Work out the finished part from the listing and answer in its coordinate system (mm). Face numbers are marked on the shaded views. A direction names the side the tool comes from. Round coordinates to 2 decimals unless told otherwise and drop trailing zeros. Write each loop counter-clockwise with the first axis right and the second up, starting at its lowest first coordinate (ties: lowest second). Pieces come first, ordered by that corner, then holes. Notation, with made-up numbers: M -12.75,55.5 L 4.25,55.5 A23 ccw 4.25,87.5 Z; hole C -32.75,-35 d8. An arc over 180 degrees is marked long. Answer in a Markdown table with one row per item.
```python
from build123d import *

# Parameters (mm, degrees)
SKETCH_W     = 100
SKETCH_H     = 70
PAD_DEPTH    = 15
PAD001_DEPTH = 10
POCKET_DEPTH = 5


with BuildPart() as part:
    # Sketch → Pad (new body)
    with BuildSketch(Plane.XY):
        Rectangle(SKETCH_W, SKETCH_H)
    extrude(amount=PAD_DEPTH)

    # Sketch001 (on Face6 of Pad) → Pad001 (join)
    with BuildSketch(Plane.XY.offset(15)):
        with BuildLine():
            Line((-37.5, -18), (-22.5, -18))
            ThreePointArc((-22.5, -18), (-16.843146, -15.656854), (-14.5, -10))
            Line((-14.5, -10), (-14.5, 10))
            ThreePointArc((-14.5, 10), (-16.843146, 15.656854), (-22.5, 18))
            Line((-22.5, 18), (-37.5, 18))
            ThreePointArc((-37.5, 18), (-43.156854, 15.656854), (-45.5, 10))
            Line((-45.5, 10), (-45.5, -10))
            ThreePointArc((-45.5, -10), (-43.156854, -15.656854), (-37.5, -18))
        make_face()
        with BuildLine():
            Line((-37.5, -15), (-22.5, -15))
            ThreePointArc((-22.5, -15), (-18.964466, -13.535534), (-17.5, -10))
            Line((-17.5, -10), (-17.5, 10))
            ThreePointArc((-17.5, 10), (-18.964466, 13.535534), (-22.5, 15))
            Line((-22.5, 15), (-37.5, 15))
            ThreePointArc((-37.5, 15), (-41.035534, 13.535534), (-42.5, 10))
            Line((-42.5, 10), (-42.5, -10))
            ThreePointArc((-42.5, -10), (-41.035534, -13.535534), (-37.5, -15))
        make_face(mode=Mode.SUBTRACT)
    pad001 = extrude(amount=PAD001_DEPTH)

    # Sketch002 (on Face5 of Pad001) → Pocket (cut)
    with BuildSketch(Plane.XY.offset(15)):
        Polygon((-25, 0), (-27.5, 4.330127), (-32.5, 4.330127), (-35, 0), (-32.5, -4.330127), (-27.5, -4.330127), align=None)
    pocket = extrude(amount=-POCKET_DEPTH, mode=Mode.SUBTRACT)

    # Mirrored: Pad001, Pocket across Sketch001 V_Axis
    add(pad001.mirror(Plane(origin=(0, 0, 15), x_dir=(0, 0, 1), z_dir=(1, 0, 0))))
    add(pocket.mirror(Plane(origin=(0, 0, 15), x_dir=(0, 0, 1), z_dir=(1, 0, 0))), mode=Mode.SUBTRACT)


solid = part.part
```
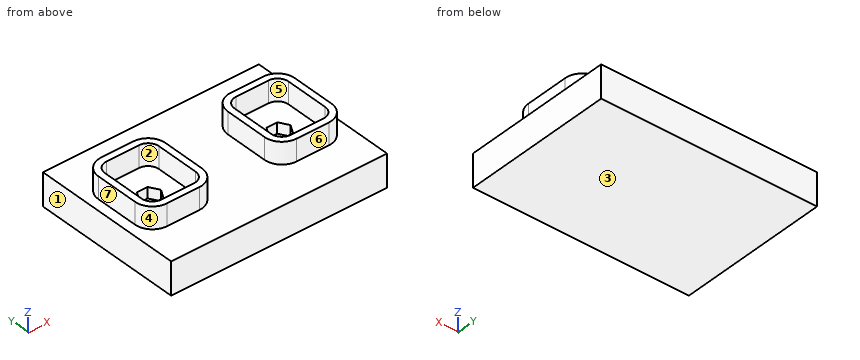
1. Given pin 1 (8 mm diameter, centred on y = -5, z = 18.5, fed in from -X); pin 2 (5 mm diameter, centred on x = -13.5, y = 16, fed in from +Z); pin 3 (3 mm diameter, centred on y = -15.5, z = 21.5, fed in from -X); pin 4 (8 mm diameter, centred on y = 4, z = 19.5, fed in from -X), each flat-ended and moving along its own axis, determine where each tip first touches the part or whether it passes through.
Calculated:
| item | result |
|---|---|
| pin 1 | stops at x = -50 |
| pin 2 | stops at z = 15 |
| pin 3 | stops at x = -44.43 |
| pin 4 | stops at x = -45.5 |
2. A tool of negligible diameter and unlimited length cuts with its end or side. For the marked faces 4, 5, 6 and 7, from which of +Z, -Z, +X, -X, +Y, -Y can it reach the whole face along a straight path? Write none if from no direction.
Calculated:
| item | result |
|---|---|
| face 4 | +Z, -X, -Y |
| face 5 | +Z |
| face 6 | +Z, +X, -X, -Y |
| face 7 | +Z, -X, +Y, -Y |
3. The part is cut by section D-D (x = 21.5). Determine the outline of the cut face in (y, z).
Calculated:
| item | result |
|---|---|
| outline | M -35,0 L 35,0 L 35,15 L 17.94,15 L 17.94,25 L 14.9,25 L 14.9,15 L -14.9,15 L -14.9,25 L -17.94,25 L -17.94,15 L -35,15 Z |
4. The part is cut by section A-A (z = 21). Count the separate pieces of the cut face and the enclosed holes in it, plus the area to 3 significant figures.
Calculated:
| item | result |
|---|---|
| separate pieces | 2 |
| enclosed holes | 2 |
| area | 665 mm² |
5. Determine the mould class of the marked faces 1, 2 and 3 for opening direction X: released by +X, released by -X, zero draft, split by the parting line, or undercut.
Calculated:
| item | result |
|---|---|
| face 1 | released by -X |
| face 2 | undercut |
| face 3 | zero draft |
6. Consider line 1 along X through (y, z) = (2.5, 22.5); line 2 along Z through (x, y) = (37, 5); line 3 along X through (y, z) = (-14, 23). Determine where each line is inside the solid, lowest interval first. Write a range as from..to.
Calculated:
| item | result |
|---|---|
| line 1 | x = -45.5..-42.5, -17.5..-14.5, 14.5..17.5, 42.5..45.5 |
| line 2 | z = 0..15 |
| line 3 | x = -44.43..-40.5, -19.5..-15.57, 15.57..19.5, 40.5..44.43 |
7. The part is cut by section B-B (z = 13.75). Determine the outline of the cut face in (x, y), plus the area to 3 significant figures.
Calculated:
| item | result |
|---|---|
| outline | M -50,-35 L 50,-35 L 50,35 L -50,35 Z; hole M -35,0 L -32.5,-4.33 L -27.5,-4.33 L -25,0 L -27.5,4.33 L -32.5,4.33 Z; hole M 25,0 L 27.5,-4.33 L 32.5,-4.33 L 35,0 L 32.5,4.33 L 27.5,4.33 Z |
| area | 6,870 mm² |
8. The part is cut by section C-C (y = -7). Determine the outline of the cut face in (x, z).
Calculated:
| item | result |
|---|---|
| outline | M -50,0 L 50,0 L 50,15 L 45.5,15 L 45.5,25 L 42.5,25 L 42.5,15 L 17.5,15 L 17.5,25 L 14.5,25 L 14.5,15 L -14.5,15 L -14.5,25 L -17.5,25 L -17.5,15 L -42.5,15 L -42.5,25 L -45.5,25 L -45.5,15 L -50,15 Z |
